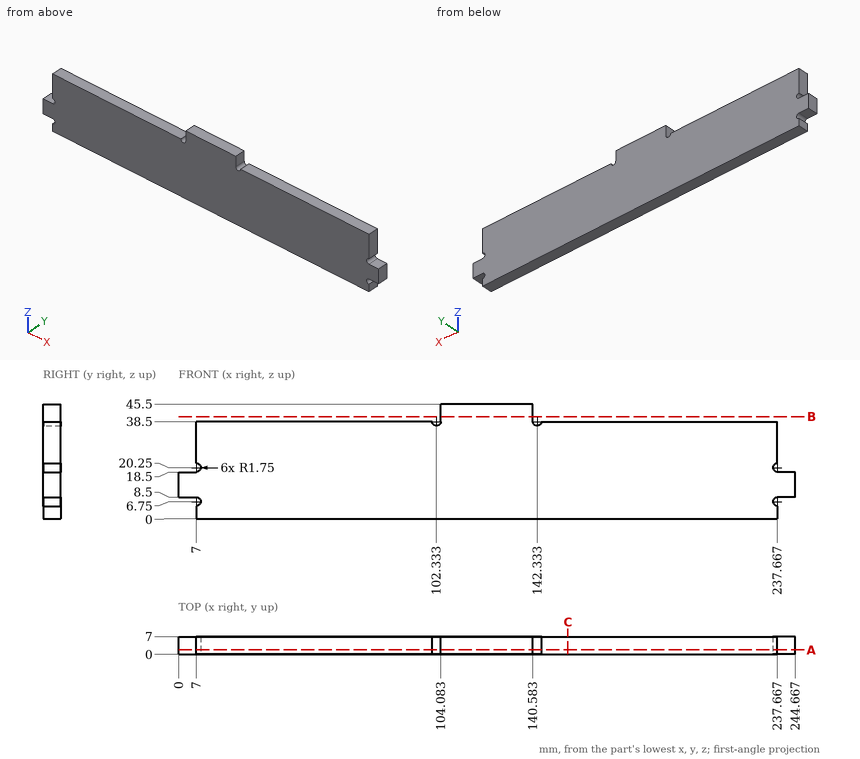
Drawing for the job (mm, zero at the part's lowest x, y, z). Give positions to 0.01 mm unless a question says otherwise; leave off trailing zeros. Order: outer loops, then holes, each group sorted by start corner. A loop starts at its lowest first (then second) coordinate and runs counter-clockwise, first axis right, second up. Notation, with made-up numbers: (28, -19) - (80, -19) arc R24 cw to (80, 17) - close; hole circle Ø7 at (26, 1). An arc over 180 degrees is marked (long way). Write item = value, one per line. Start each with the question number.
1. Probe line 1 along Z through (x, y) = (233.5, 6.75); line 2 along X through (y, z) = (1, 42); line 3 along X through (y, z) = (3.5, 24). List the from-to ranges inside material, lowest first.
2. Cut at A-A, the plane y = 1.75. List the corners of the cut face in (x, z).
3. Cut at B-B, the plane z = 40.5. List the corners of the cut face in (x, y).
4. Drop flat-ended pins along their axis: P1, Ø2.5, axis at y = 3, z = 1.5, coming from the +X side; P2, Ø3.5, axis at y = 3.5, z = 41.5, coming from the -X side; P3, Ø3.5, axis at x = 241.5, y = 5, coming from the +Z side. Give the stop position or say it passes through.
5. Cut at C-C, the plane x = 154.5. List the corners of the cut face in (y, z).
Taken from the geometry:
q1.line_1 = 0 to 38.5
q1.line_2 = 104.08 to 140.58
q1.line_3 = 7 to 237.67
q2.outline = (0, 8.5) - (7, 8.5) arc R1.75 cw to (7, 5) - (7, 0) - (237.67, 0) - (237.67, 5) arc R1.75 cw to (237.67, 8.5) - (244.67, 8.5) - (244.67, 18.5) - (237.67, 18.5) arc R1.75 cw to (237.67, 22) - (237.67, 38.5) - (144.08, 38.5) arc R1.75 cw to (140.58, 38.5) - (140.58, 45.5) - (104.08, 45.5) - (104.08, 38.5) arc R1.75 cw to (100.58, 38.5) - (7, 38.5) - (7, 22) arc R1.75 cw to (7, 18.5) - (0, 18.5) - close
q3.outline = (104.08, 0) - (140.58, 0) - (140.58, 7) - (104.08, 7) - close
q4.P1 = 237.67
q4.P2 = 104.08
q4.P3 = 18.5
q5.outline = (0, 0) - (7, 0) - (7, 38.5) - (0, 38.5) - close
